Verification items for the finished model (mm, model axes). Face numbers are marked on the shaded views. A direction names the side the tool comes from. Coordinates: 2 decimals unless noted, no trailing zeros. Order: outer loops, then holes, each group sorted by start corner. A loop starts at its lowest first (then second) coordinate and runs counter-clockwise, first axis right, second up. Notation, with made-up numbers: (20, 16.25) -> (41, 16.25) arc R20 cw to (41, 49.25) -> close; hole circle Ø11 at (75, 80.25). An arc over 180 degrees is marked (long way). Answer as CSV lines item,"result".
```python
from build123d import *

# Parameters (mm, degrees)
SKETCH2_W           = 94
SKETCH2_H           = 59.5
BOSS_EXTRUDE1_DEPTH = 11
SKETCH3_W           = 90
SKETCH3_H           = 55.5
CUT_EXTRUDE1_DEPTH  = 9
SKETCH5_W           = 6
SKETCH5_H           = 59.5
CUT_EXTRUDE2_DEPTH  = 2


with BuildPart() as part:
    # Sketch2 → Boss-Extrude1 (new body)
    with BuildSketch(Plane.XY):
        Rectangle(SKETCH2_W, SKETCH2_H)
    extrude(amount=BOSS_EXTRUDE1_DEPTH)

    # Sketch3 → Cut-Extrude1 (cut)
    with BuildSketch(Plane.XY.offset(11)):
        Rectangle(SKETCH3_W, SKETCH3_H)
    extrude(amount=-CUT_EXTRUDE1_DEPTH, mode=Mode.SUBTRACT)

    # Sketch5 → Cut-Extrude2 (cut)
    with BuildSketch(Plane(origin=(0, 0, 0), x_dir=(-1, 0, 0), z_dir=(0, 0, -1))):
        with Locations((-42, 0)):
            Rectangle(SKETCH5_W, SKETCH5_H)
    extrude(amount=-CUT_EXTRUDE2_DEPTH, mode=Mode.SUBTRACT)


solid = part.part
```
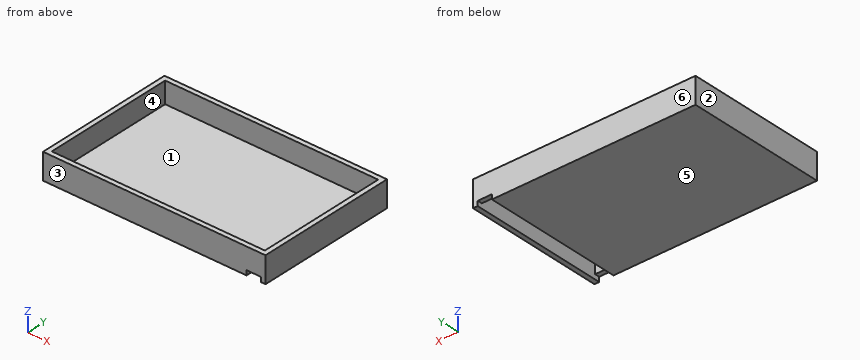
Item 1: Section check A-A, the plane y = -23. Record the boundary of the cut face in (x, z).
Answer list:
outline,"(-47, 0) -> (39, 0) -> (39, 2) -> (-45, 2) -> (-45, 11) -> (-47, 11) -> close; (45, 0) -> (47, 0) -> (47, 11) -> (45, 11) -> close"
Item 2: Section check C-C, the plane z = 9. Record the boundary of the cut face in (x, y).
Answer list:
outline,"(-47, -29.75) -> (47, -29.75) -> (47, 29.75) -> (-47, 29.75) -> close; hole (-45, -27.75) -> (45, -27.75) -> (45, 27.75) -> (-45, 27.75) -> close"
Item 3: Thickness scan on line 1 (X direction, y = -6.5, z = 5.75); line 2 (Y direction, x = -33, z = 3); line 3 (X direction, y = -16, z = 1.5). Record the ranges inside material, lowest first.
Answer list:
line 1,"-47 to -45, 45 to 47"
line 2,"-29.75 to -27.75, 27.75 to 29.75"
line 3,"-47 to 39, 45 to 47"
Item 4: Depth check by flat-ended pin: pin 1 Ø1 at (x, y) = (43, 29) entering from -Z; pin 2 Ø10 at (x, y) = (-36, 16.5) entering from +Z. Enter the tip coordinate at first touch or a pass-through.
Answer list:
pin 1,"z = 2"
pin 2,"z = 2"
Item 5: Release check for a two-part mould opening along Y. For the marked faces 3, 4, 5 and 6 record: +Y half, -Y half, draft (parallel to the pull), parting line (faces both ways), or undercut.
Answer list:
face 3,"-Y half"
face 4,"undercut"
face 5,"draft"
face 6,"+Y half"
Item 6: Section check B-B, the plane x = -17. Record the boundary of the cut face in (y, z), plus the area to 3 significant figures.
Answer list:
outline,"(-29.75, 0) -> (29.75, 0) -> (29.75, 11) -> (27.75, 11) -> (27.75, 2) -> (-27.75, 2) -> (-27.75, 11) -> (-29.75, 11) -> close"
area,"155 mm2"
Item 7: Tool access check on the marked faces 1 and 2. Record the directions out of +Z, -Z, +X, -X, +Y, -Y that give a thin tool (end or side, any length) a straight path to the whole face; none if there is none.
Answer list:
face 1,"+Z"
face 2,"+Z, -Z, -X, +Y, -Y"
